Part print with two shaded views. Sizes in mm from the minimum x, y, z corner. Round coordinates to 2 decimals unless told otherwise and drop trailing zeros. Loops run counter-clockwise (first coordinate to the right, second up) from the corner with the lowest first, then second, coordinate; pieces in that order, holes last. Notation, with made-up numbers: (41, 50) -> (72, 50) arc R25 cw to (72, 66) -> close; hole circle Ø10 at (38, -28). An arc over 180 degrees is marked (long way). Use a Markdown table: item, result. Add a question column.
Item 1: Cut at A-A, the plane x = 20.5. List the corners of the cut face in (y, z).
Item 2: Flat gauge pins, fed straight in: pin 1 (1.7 mm diameter, centred on y = 18.5, z = 17.5, fed in from +X); pin 2 (1.7 mm diameter, centred on x = 138.5, z = 16.5, fed in from -Y); pin 3 (2.5 mm diameter, centred on y = 31.5, z = 16.5, fed in from -X). Where does each tip first touch, or does it go through?
Item 3: Probe line 1 (X direction, y = 30.3, z = 4.25); line 2 (Y direction, x = 198, z = 4); line 3 (Y direction, x = 155.5, z = 16.5). List the from-to ranges inside material, lowest first. Write a range as [from, to].
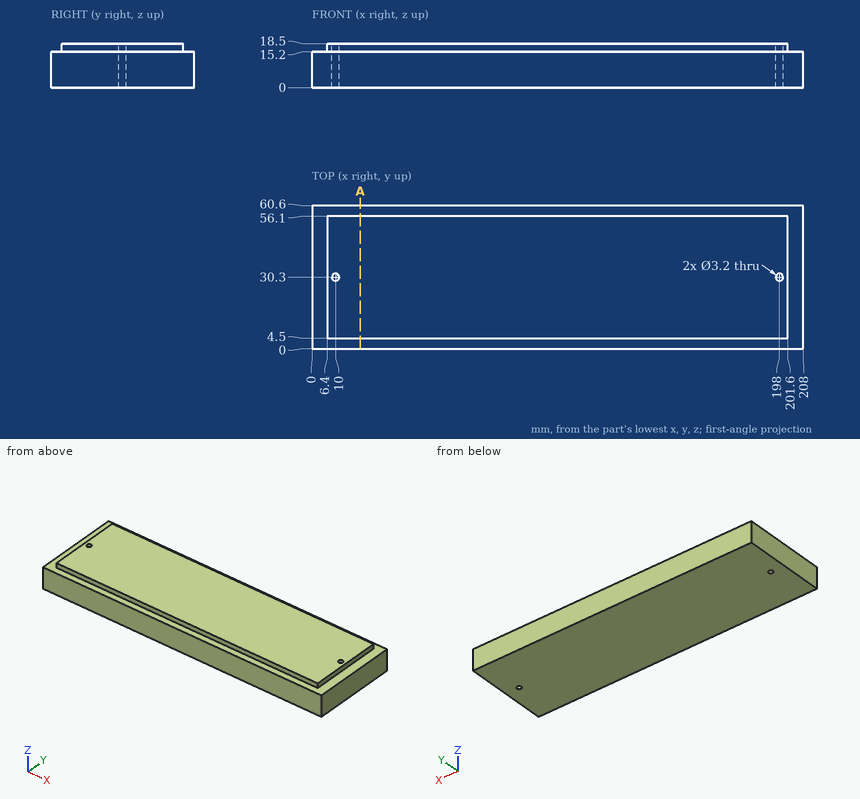
A:
| question | item | result |
|---|---|---|
| 1 | outline | (0, 0) -> (60.6, 0) -> (60.6, 15.2) -> (56.1, 15.2) -> (56.1, 18.5) -> (4.5, 18.5) -> (4.5, 15.2) -> (0, 15.2) -> close |
| 2 | pin 1 | stops at x = 201.6 |
| 2 | pin 2 | stops at y = 4.5 |
| 2 | pin 3 | stops at x = 6.4 |
| 3 | line 1 | x = [0, 8.4], [11.6, 196.4], [199.6, 208] |
| 3 | line 2 | y = [0, 28.7], [31.9, 60.6] |
| 3 | line 3 | y = [4.5, 56.1] |
